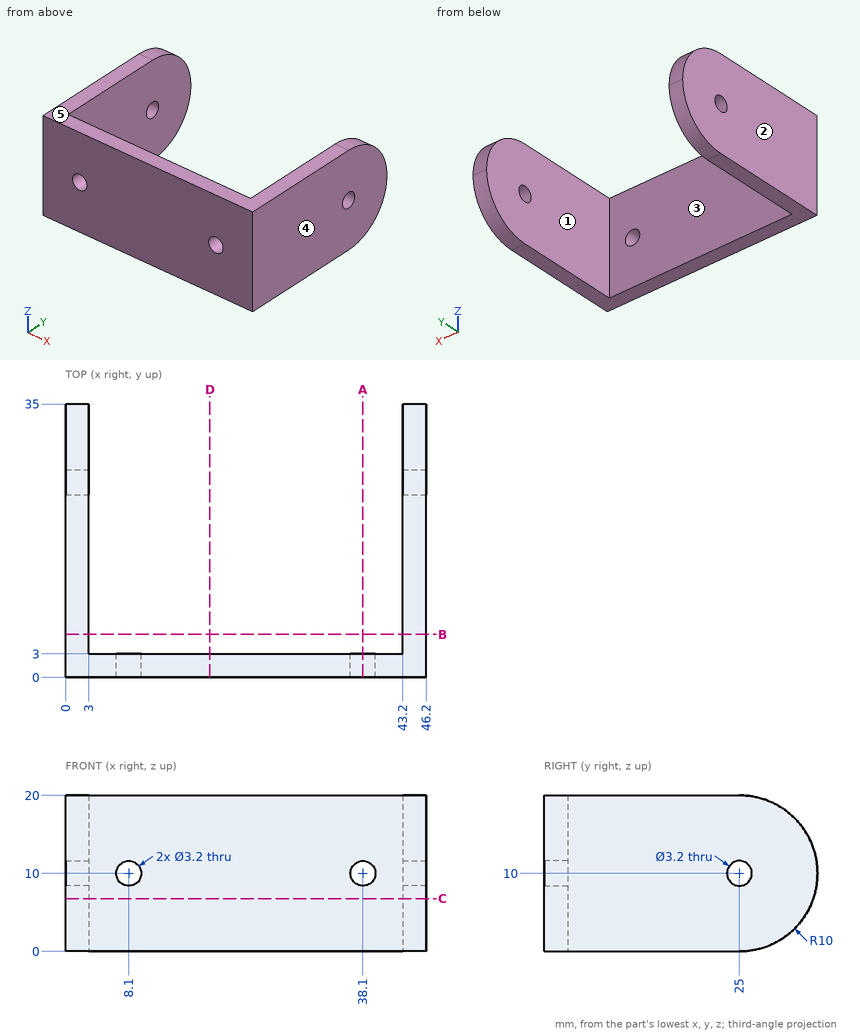
Geometry: see drawing. Coordinates: mm, zero at the bounding-box minimum. A direction names the side the tool comes from. Coordinates: 2 decimals unless noted, no trailing zeros. Loops run counter-clockwise (first coordinate to the right, second up) from the corner with the lowest first, then second, coordinate; pieces in that order, holes last.
Q1. Cut plane B-B (y = 5.5). Output: boundary loops of the cut face in (x, z).
Q2. Material intervals for line 1 (X direction, y = 1.3, z = 10); line 2 (X direction, y = 32, z = 9); line 3 (Y direction, x = 1.55, z = 10), sorted ascending.
Q3. Set-up query: the marked faces 1 and 2. Return all of +Z, -Z, +X, -X, +Y, -Y with unobstructed straight access to the full face (end or side cutting, diameter ignored); none if empty.
Q4. Cut plane D-D (x = 18.5). Output: boundary loops of the cut face in (y, z).
Q5. Draft query along X for the marked faces 3, 4 and 5. Return one class per face: +X half, -X half, draft (parallel to the pull), parting line (faces both ways), or undercut.
Q6. Cut plane A-A (x = 38.1). Output: boundary loops of the cut face in (y, z).
Q7. Contact query for flat-ended pins moving along their axis: pin 1 (3 mm diameter, centred on x = 24.5, z = 12.5, fed in from +Y); pin 2 (4 mm diameter, centred on y = 29.5, z = 13, fed in from -X). Output: stop coordinate, or through.
Q8. Cut plane C-C (z = 6.75). Output: boundary loops of the cut face in (x, y).
Working result:
1. outline: (0, 0) - (3, 0) - (3, 20) - (0, 20) - close; (43.2, 0) - (46.2, 0) - (46.2, 20) - (43.2, 20) - close
2. line 1: x = 0 to 6.5, 9.7 to 36.5, 39.7 to 46.2
2. line 2: x = 0 to 3, 43.2 to 46.2
2. line 3: y = 0 to 23.4, 26.6 to 35
3. face 1: +Z, -Z, +Y
3. face 2: +Z, -Z, -X, +Y, -Y
4. outline: (0, 0) - (3, 0) - (3, 20) - (0, 20) - close
5. face 3: undercut
5. face 4: +X half
5. face 5: draft
6. outline: (0, 0) - (3, 0) - (3, 8.4) - (0, 8.4) - close; (0, 11.6) - (3, 11.6) - (3, 20) - (0, 20) - close
7. pin 1: stops at y = 3
7. pin 2: stops at x = 0
8. outline: (0, 0) - (46.2, 0) - (46.2, 34.46) - (43.2, 34.46) - (43.2, 3) - (3, 3) - (3, 34.46) - (0, 34.46) - close
